from build123d import *

# Parameters (mm, degrees)
SKETCH1_W           = 55
SKETCH1_H           = 19
BOSS_EXTRUDE1_DEPTH = 1.5
SKETCH2_R           = 1.675
CUT_EXTRUDE1_DEPTH  = 1.5
SKETCH3_W           = 2.95
SKETCH3_H           = 3.35
BOSS_EXTRUDE2_DEPTH = 1.6


with BuildPart() as part:
    # Sketch1 → Boss-Extrude1 (new body)
    with BuildSketch(Plane.XY):
        Rectangle(SKETCH1_W, SKETCH1_H)
    extrude(amount=BOSS_EXTRUDE1_DEPTH)

    # Sketch2 → Cut-Extrude1 (cut)
    with BuildSketch(Plane.XY.offset(1.5)):
        with Locations((-24.475, 5.075)):
            Circle(SKETCH2_R)
        with Locations((24.475, 5.075)):
            Circle(SKETCH2_R)
    extrude(amount=-CUT_EXTRUDE1_DEPTH, mode=Mode.SUBTRACT)

    # Sketch3 → Boss-Extrude2 (add)
    with BuildSketch(Plane.XY.offset(1.5)):
        with Locations((-0.625, 2.545)):
            Rectangle(SKETCH3_W, SKETCH3_H)
        with Locations((20.825, -2.605)):
            Rectangle(SKETCH3_W, SKETCH3_H)
        with Locations((-20.825, -2.605)):
            Rectangle(SKETCH3_W, SKETCH3_H)
    extrude(amount=BOSS_EXTRUDE2_DEPTH)


solid = part.part
Check sheet for the modelled part. Datum: model origin and axes. Units: mm. A direction names the side the tool comes from. Round coordinates to 2 decimals unless told otherwise and drop trailing zeros. Loops run counter-clockwise (first coordinate to the right, second up) from the corner with the lowest first, then second, coordinate; pieces in that order, holes last. Notation, with made-up numbers: M 72,55.5 L 79,55.5 A12 cw 79,62.5 Z; hole C -10.75,-0.5 d8. An arc over 180 degrees is marked long. One line per item, written item: value.
(1) Sectioned sample at B-B, the plane x = -20. Record the cut outline in (y, z).
Computed values:
outline: M -9.5,0 L 9.5,0 L 9.5,1.5 L -0.93,1.5 L -0.93,3.1 L -4.28,3.1 L -4.28,1.5 L -9.5,1.5 Z
(2) Depth check by flat-ended pin: pin 1 Ø1.8 at (y, z) = (3, 2.5) entering from -X; pin 2 Ø0.8 at (y, z) = (-2, 2.5) entering from +X; pin 3 Ø0.8 at (x, z) = (0, 2.5) entering from +Y; pin 4 Ø1.3 at (x, z) = (-1, 2) entering from -Y. Enter the tip coordinate at first touch or a pass-through.
Computed values:
pin 1: stops at x = -2.1
pin 2: stops at x = 22.3
pin 3: stops at y = 4.22
pin 4: stops at y = -9.5
(3) Access from +Z, -Z, +X, -X, +Y, -Y to the whole of each face (thin tool, end or side, straight path). Record for faces 4 (the face through (-19.35, -3, 2)), 5 (the face through (0.85, 3, 2)), 6 (the face through (-22.3, -3, 2)).
Computed values:
face 4: +Z, +Y, -Y
face 5: +Z, +X, +Y, -Y
face 6: +Z, -X, +Y, -Y
(4) Sectioned sample at C-C, the plane y = -7.5. Record the cut outline in (x, z), then the cut area to 3 significant figures.
Computed values:
outline: M -27.5,0 L 27.5,0 L 27.5,1.5 L -27.5,1.5 Z
area: 82.5 mm^2
(5) Sectioned sample at A-A, the plane z = 2.5. Record the cut outline in (x, y).
Computed values:
outline: M -22.3,-4.28 L -19.35,-4.28 L -19.35,-0.93 L -22.3,-0.93 Z; M -2.1,0.87 L 0.85,0.87 L 0.85,4.22 L -2.1,4.22 Z; M 19.35,-4.28 L 22.3,-4.28 L 22.3,-0.93 L 19.35,-0.93 Z
(6) Sectioned sample at D-D, the plane x = 14.5. Record the cut outline in (y, z).
Computed values:
outline: M -9.5,0 L 9.5,0 L 9.5,1.5 L -9.5,1.5 Z
(7) Release check for a two-part mould opening along Y. For faces 1 (the face through (21, -4.28, 2)), 2 (the face through (0, 9.5, 1)), 3 (the face through (-22.93, 4.43, 0.76)) record: +Y half, -Y half, draft (parallel to the pull), parting line (faces both ways), or undercut.
Computed values:
face 1: -Y half
face 2: +Y half
face 3: undercut
(8) Thickness scan on line 1 (X direction, y = 6.25, z = 0.2); line 2 (X direction, y = -4.25, z = 1.7); line 3 (Z direction, x = 8.5, y = -1). Record the ranges inside material, lowest first.
Computed values:
line 1: x = -27.5 to -25.67, -23.28 to 23.28, 25.67 to 27.5
line 2: x = -22.3 to -19.35, 19.35 to 22.3
line 3: z = 0 to 1.5
